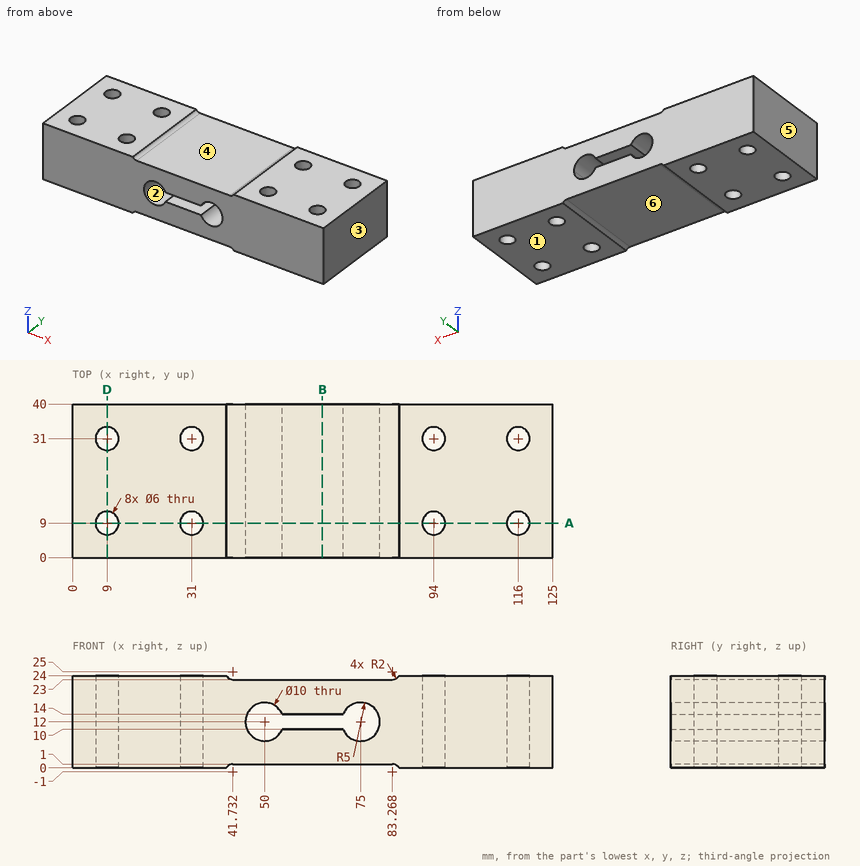
Print and shaded views of the part. All mm, measured from the part's lowest x, y and z. A direction names the side the tool comes from. Round coordinates to 2 decimals unless told otherwise and drop trailing zeros. Write each loop counter-clockwise with the first axis right and the second up, starting at its lowest first coordinate (ties: lowest second). Pieces come first, ordered by that corner, then holes. Notation, with made-up numbers: (74, -29) -> (131, -29) arc R22 cw to (131, -1) -> close; hole circle Ø6 at (59.5, -25.5). An arc over 180 degrees is marked (long way). Write item = value, one per line.
(1) Band-saw the part on D-D (x = 9). Give the cut face in (y, z).
Answer:
outline = (0, 0) -> (6, 0) -> (6, 24) -> (0, 24) -> close; (12, 0) -> (28, 0) -> (28, 24) -> (12, 24) -> close; (34, 0) -> (40, 0) -> (40, 24) -> (34, 24) -> close
(2) Flat gauge pins, fed straight in: pin 1 (11.5 mm diameter, centred on x = 50, z = 12, fed in from -Y); pin 2 (6 mm diameter, centred on x = 54, y = 8, fed in from -Z); pin 3 (20 mm diameter, centred on x = 71.5, y = 21.5, fed in from +Z). Where does each tip first touch, or does it go through?
Answer:
pin_1 = 0
pin_2 = 1
pin_3 = 23
(3) Two-plate mould, pull along X, no slides. Class the marked faces 1, 2 and 3: pulls with the +X half, pulls with the -X half, needs draft (parallel to the pull), parting line crosses it, or undercut.
Answer:
face_1 = needs draft
face_2 = undercut
face_3 = pulls with the +X half
(4) Band-saw the part on B-B (x = 65). Give the cut face in (y, z).
Answer:
outline = (0, 1) -> (40, 1) -> (40, 10) -> (0, 10) -> close; (0, 14) -> (40, 14) -> (40, 23) -> (0, 23) -> close
(5) Band-saw the part on A-A (y = 9). State how many separate pieces and enclosed holes the cut face has, then the cut area to 3 significant figures.
Answer:
separate_pieces = 5
enclosed_holes = 1
area = 2,120 mm2
(6) Probe L1, parallel to Y at x = 116, z = 7.75; L2, parallel to X at y = 20.5, z = 14.5; L3, parallel to X at y = 17, z = 12. List the from-to ranges inside material, lowest first.
Answer:
L1 = 0 to 6, 12 to 28, 34 to 40
L2 = 0 to 45.67, 54.33 to 70.67, 79.33 to 125
L3 = 0 to 45, 80 to 125
(7) Tool access for the marked faces 4, 5 and 6: list every direction of +Z, -Z, +X, -X, +Y, -Y with a clear straight run to the whole face (end or side of a thin tool).
Answer:
face_4 = +Z, +Y, -Y
face_5 = +Z, -Z, -X, +Y, -Y
face_6 = -Z, +Y, -Y
